```python
from build123d import *

# Parameters (mm, degrees)
SKETCH1_W           = 92.7
SKETCH1_H           = 227
BOSS_EXTRUDE1_DEPTH = 3
SKETCH3_R           = 2
CUT_EXTRUDE1_DEPTH  = 4
FILLET1_R           = 10


with BuildPart() as part:
    # Sketch1 → Boss-Extrude1 (new body)
    with BuildSketch(Plane(origin=(0, 0, 0), x_dir=(1, 0, 0), z_dir=(0, 1, 0))):
        with Locations((0, -3.5)):
            Rectangle(SKETCH1_W, SKETCH1_H)
    extrude(amount=BOSS_EXTRUDE1_DEPTH)

    # Sketch3 → Cut-Extrude1 (cut, through all)
    with BuildSketch(Plane.XZ):
        Polygon((-46.35, -110), (-45.148132032, -110), (-32.56577351, -87.57595075), (-46.35, -66.656688952), align=None)
        Polygon((-46.35, -41.75), (-46.35, -66.315996364), (-32.56577351, -41.75), align=None)
        with Locations((-30.338884711, -100)):
            Circle(SKETCH3_R)
        with Locations((-14.338884711, -97)):
            Circle(SKETCH3_R)
        Polygon((32.565746646, -91.25), (4.338884711, -91.25), (4.338884711, -110), (46.35, -110), (46.35, -66.68400328), align=None)
        Polygon((32.766055192, -45.29151818), (46.35, -66.340018534), (46.35, -21.082506998), align=None)
        with Locations((30.338884711, -33)):
            Circle(SKETCH3_R)
        with Locations((14.338884711, -36)):
            Circle(SKETCH3_R)
        with Locations((14.338884711, -81.25)):
            Circle(SKETCH3_R)
        Polygon((-46.35, 117), (-46.35, 73.684003636), (-32.56577351, 98.25), (-4.338884711, 98.25), (-4.338884711, 117), align=None)
        Polygon((-46.35, 73.343311048), (-46.35, 27.858052887), (-32.56577351, 52.42404925), align=None)
        Polygon((32.565746646, 48.75), (46.35, 48.75), (46.35, 73.31599672), align=None)
        Polygon((32.766055192, 94.70848182), (46.35, 73.659981466), (46.35, 117), (45.274073399, 117), align=None)
        with Locations((14.338884711, 58.75)):
            Circle(SKETCH3_R)
        with Locations((14.338884711, 104)):
            Circle(SKETCH3_R)
        with Locations((30.338884711, 107)):
            Circle(SKETCH3_R)
        with Locations((-14.338884711, 43)):
            Circle(SKETCH3_R)
        with Locations((-30.338884711, 40)):
            Circle(SKETCH3_R)
        with Locations((-14.338884711, 88.25)):
            Circle(SKETCH3_R)
        with Locations((-14.338884711, -51.75)):
            Circle(SKETCH3_R)
    extrude(amount=-CUT_EXTRUDE1_DEPTH, mode=Mode.SUBTRACT)

    # Fillet1
    fillet1_edges = [part.edges().sort_by_distance(p)[0] for p in [
        (46.35, 1.5, 48.75),
        (-4.338884711, 1.5, 117),
        (4.338884711, 1.5, -110),
        (-46.35, 1.5, -41.75),
    ]]
    fillet(fillet1_edges, radius=FILLET1_R)


solid = part.part
```
Geometry: final body of the model. Coordinates: model frame, mm. A direction names the side the tool comes from. Round coordinates to 2 decimals unless told otherwise and drop trailing zeros. Write each loop counter-clockwise with the first axis right and the second up, starting at its lowest first coordinate (ties: lowest second). Pieces come first, ordered by that corner, then holes. Notation, with made-up numbers: (81, 54.5) -> (110, 54.5) arc R13 ccw to (110, 58.5) -> close; hole circle Ø5 at (63.25, 72). An arc over 180 degrees is marked (long way). Return JSON: item names as keys, results as strings.
Q1. Set-up query: faces 5 (the flat face through (39.463, 1.479, 84.332)), 6 (the flat face through (-39.361, 1.479, -77.263)), 7 (the cylindrical face through (-14.599, 1.479, -95.017)). Return all of +Z, -Z, +X, -X, +Y, -Y with unobstructed straight access to the full face (end or side cutting, diameter ignored); none if empty.
From the geometry:
{"face 5": "+X, +Y, -Y", "face 6": "-X, +Y, -Y", "face 7": "+Y, -Y"}
Q2. First-contact query: pin 1 Ø3.5 at (x, z) = (30.34, -33) entering from -Y; pin 2 Ø1.5 at (y, z) = (2, 101) entering from -X; pin 3 Ø1 at (y, z) = (1.5, 30.5) entering from -X. Flat tips, straight axial feed; report the tip coordinate or a pass-through.
From the geometry:
{"pin 1": "through", "pin 2": "x = -4.34", "pin 3": "x = -45.15"}
Q3. Mould query, pull axis X, two halves, no side actions, for faces 1 (the cylindrical face through (1.33, 1.52, -107.15)), 2 (the flat face through (-1, 0, 2)), 3 (the cylindrical face through (14.079, 1.479, 105.983)), 4 (the cylindrical face through (-14.599, 1.479, 90.233)). Classes: +X half, -X half, draft (parallel to the pull), parting line (faces both ways), or undercut.
From the geometry:
{"face 1": "+X half", "face 2": "draft", "face 3": "undercut", "face 4": "undercut"}
Q4. Section A-A on z = -81.25. Return the cut outline in (x, y), and give its area (3 significant figures).
From the geometry:
{"outline": "(-36.73, 0) -> (12.34, 0) -> (12.34, 3) -> (-36.73, 3) -> close; (16.34, 0) -> (38.18, 0) -> (38.18, 3) -> (16.34, 3) -> close", "area": "213 mm2"}
Q5. Ray query, line 1 (Z direction, x = -14, y = 0.9); line 2 (Z direction, x = -38, y = 1.5); line 3 (Z direction, x = 16, y = 1.4). Return the intervals inside material, ascending.
From the geometry:
{"line 1": "-110 to -98.97, -95.03 to -53.72, -49.78 to 41.03, 44.97 to 86.28, 90.22 to 98.25", "line 2": "-110 to -97.26, -79.33 to -51.43, -41.61 to 42.74, 60.67 to 88.57", "line 3": "-91.25 to -82.36, -80.14 to -37.11, -34.89 to 57.64, 59.86 to 102.89, 105.11 to 117"}
Q6. Section B-B on y = 1.9. Give the number of separate pieces and of enclosed holes in the cut face, and give its area (3 significant figures).
From the geometry:
{"separate pieces": "1", "enclosed holes": "12", "area": "17,300 mm2"}
Q7. Section C-C on z = 88.25. Return the cut outline in (x, y).
From the geometry:
{"outline": "(-38.18, 0) -> (-16.34, 0) -> (-16.34, 3) -> (-38.18, 3) -> close; (-12.34, 0) -> (36.93, 0) -> (36.93, 3) -> (-12.34, 3) -> close"}
